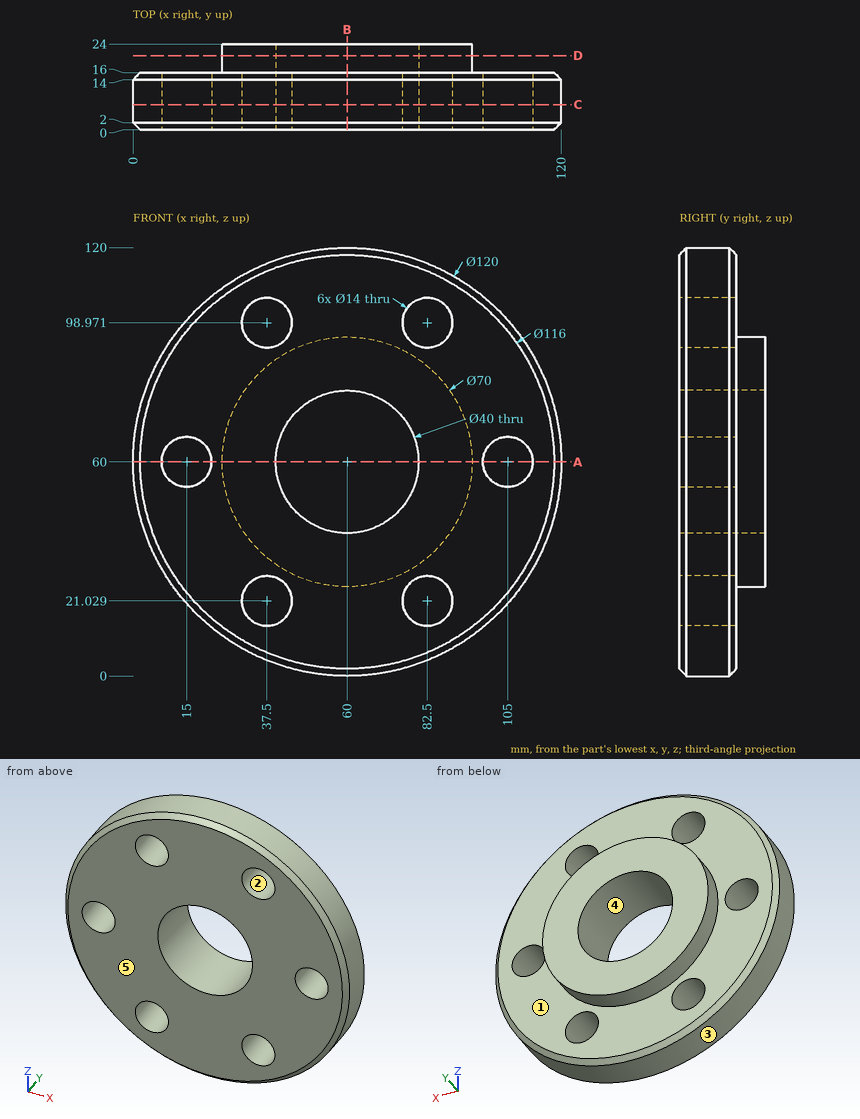
The drawing under review shows one solid part. Ordinate dimensions are in mm from its lowest x, y, z. A direction names the side the tool comes from. Round coordinates to 2 decimals unless told otherwise and drop trailing zeros. Write each loop counter-clockwise with the first axis right and the second up, starting at its lowest first coordinate (ties: lowest second). Pieces come first, ordered by that corner, then holes. Notation, with made-up numbers: (36.25, 78.5) - (88.25, 78.5) arc R22 ccw to (88.25, 95.5) - close; hole circle Ø2 at (-26.75, 78.25). An arc over 180 degrees is marked (long way). Use a Markdown table: item, result. Add a question column.
1. We need section A-A (z = 60). State the section outline as (x, y) points.
2. Mouldability with a two-part tool opening along Z and no side actions: class the marked faces 3, 4 and 5 as +Z half, -Z half, draft (parallel to the pull), parting line (faces both ways), or undercut.
3. We need section C-C (y = 7). State the section outline as (x, z) points.
4. Wall thickness on probe 1 along Z at (x, y) = (61, 22.5) (1 decimal); probe 2 along X at (y, z) = (5.5, 22); probe 3 along X at (y, z) = (4.5, 22.5): over which ranges is each line inside the solid? List them lowest first.
5. For the marked faces 1 and 2, list the 3-axis set-ups (+Z, -Z, +X, -X, +Y, -Y) from which the entire face can be reached by the end or side of a thin tool; tool diameter is ignored.
6. Clearance check with flat-ended pins moving along their axes: pin 1 (6 mm diameter, centred on x = 15.5, z = 40.5, fed in from +Y); pin 2 (8.5 mm diameter, centred on x = 105, z = 60, fed in from -Y) (3 decimals); pin 3 (8 mm diameter, centred on y = 12.5, z = 107, fed in from +X) (1 decimal); pin 4 (2 mm diameter, centred on y = 12.5, z = 107, fed in from +X). State where each tip first meets the part, or that it passes through.
7. We need section B-B (x = 60). State the section outline as (y, z) points.
8. We need section D-D (y = 20.75). State the section outline as (x, z) points.
Output:
| question | item | result |
|---|---|---|
| 1 | outline | (0, 2) - (2, 0) - (8, 0) - (8, 16) - (2, 16) - (0, 14) - close; (22, 0) - (40, 0) - (40, 24) - (25, 24) - (25, 16) - (22, 16) - close; (80, 0) - (98, 0) - (98, 16) - (95, 16) - (95, 24) - (80, 24) - close; (112, 0) - (118, 0) - (120, 2) - (120, 14) - (118, 16) - (112, 16) - close |
| 2 | face 3 | parting line |
| 2 | face 4 | undercut |
| 2 | face 5 | draft |
| 3 | outline | circle Ø120 at (60, 60); hole circle Ø14 at (15, 60); hole circle Ø14 at (37.5, 21.03); hole circle Ø14 at (37.5, 98.97); hole circle Ø40 at (60, 60); hole circle Ø14 at (82.5, 21.03); hole circle Ø14 at (82.5, 98.97); hole circle Ø14 at (105, 60) |
| 4 | probe 1 | z = 25 to 40, 80 to 95 |
| 4 | probe 2 | x = 13.57 to 30.57, 44.43 to 75.57, 89.43 to 106.43 |
| 4 | probe 3 | x = 13.16 to 30.66, 44.34 to 75.66, 89.34 to 106.84 |
| 5 | face 1 | +Y |
| 5 | face 2 | +Y, -Y |
| 6 | pin 1 | stops at y = 16 |
| 6 | pin 2 | passes through |
| 6 | pin 3 | stops at x = 101.8 |
| 6 | pin 4 | stops at x = 98.52 |
| 7 | outline | (0, 2) - (2, 0) - (14, 0) - (16, 2) - (16, 25) - (24, 25) - (24, 40) - (0, 40) - close; (0, 80) - (24, 80) - (24, 95) - (16, 95) - (16, 118) - (14, 120) - (2, 120) - (0, 118) - close |
| 8 | outline | circle Ø70 at (60, 60); hole circle Ø40 at (60, 60) |
